Input: part model. Units: mm. Frame: model coordinates. Coordinates: 2 decimals unless noted, no trailing zeros. Loops run counter-clockwise (first coordinate to the right, second up) from the corner with the lowest first, then second, coordinate; pieces in that order, holes last.
(1) Section A-A, the plane z = 1.3. Return loops of the section in (x, y).
(2) Section C-C, the plane y = 17.5. Return loops of the section in (x, z), then the cut area to 3 significant figures.
(3) Section B-B, the plane x = -32.5. Return loops of the section in (y, z), then the cut area to 3 significant figures.
(4) Line query: L1, parallel to Y at x = -23, z = 0.3; L2, parallel to X at y = 19, z = 2.1; L3, parallel to X at y = 17.25, z = 1.9. Output: solid intervals per line, ascending.
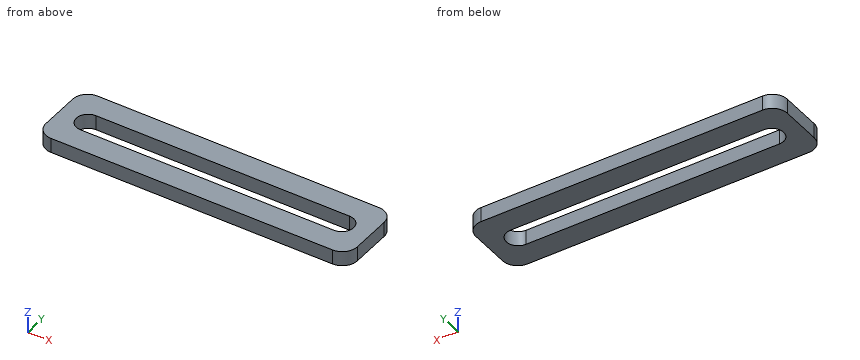
```python
from build123d import *

# Parameters (mm, degrees)
F0_W     = 53
F0_H     = 12
F1_DEPTH = 2.5
F2_R     = 2.54


with BuildPart() as f1:
    # F0 (on Top) → F1 (new body)
    with BuildSketch(Plane.XY):
        with Locations((-32.425053, 18.900206)):
            Rectangle(F0_W, F0_H)
        with BuildLine():
            Line((-54.015053, 20.900206), (-10.835053, 20.900206))
            ThreePointArc((-10.835053, 20.900206), (-8.835053, 18.900206), (-10.835053, 16.900206))
            Line((-10.835053, 16.900206), (-54.015053, 16.900206))
            ThreePointArc((-54.015053, 16.900206), (-56.015053, 18.900206), (-54.015053, 20.900206))
        make_face(mode=Mode.SUBTRACT)
    extrude(amount=F1_DEPTH)

    # F2
    f2_edges = [f1.edges().sort_by_distance(p)[0] for p in [
        (-58.925053, 24.900206, 1.25),
        (-58.925053, 12.900206, 1.25),
        (-5.925053, 12.900206, 1.25),
        (-5.925053, 24.900206, 1.25),
    ]]
    fillet(f2_edges, radius=F2_R)


solid = f1.part
```
Report:
1. outline: (-58.93, 15.44) arc R2.54 ccw to (-56.39, 12.9) - (-8.47, 12.9) arc R2.54 ccw to (-5.93, 15.44) - (-5.93, 22.36) arc R2.54 ccw to (-8.47, 24.9) - (-56.39, 24.9) arc R2.54 ccw to (-58.93, 22.36) - close; hole (-54.02, 16.9) - (-10.84, 16.9) arc R2 ccw to (-10.84, 20.9) - (-54.02, 20.9) arc R2 ccw to start
2. outline: (-58.93, 0) - (-55.44, 0) - (-55.44, 2.5) - (-58.93, 2.5) - close; (-9.41, 0) - (-5.93, 0) - (-5.93, 2.5) - (-9.41, 2.5) - close
2. area: 17.4 mm2
3. outline: (12.9, 0) - (16.9, 0) - (16.9, 2.5) - (12.9, 2.5) - close; (20.9, 0) - (24.9, 0) - (24.9, 2.5) - (20.9, 2.5) - close
3. area: 20.0 mm2
4. L1: y = 12.9 to 16.9, 20.9 to 24.9
4. L2: x = -58.93 to -56.01, -8.84 to -5.93
4. L3: x = -58.93 to -55.15, -9.71 to -5.93
